```python
from build123d import *

# Parameters (mm, degrees)
F0_R      = 32.5
F1_DEPTH  = 196
F2_SIZE2  = 0.5
F2_SIZE   = 26
F3_R      = 32
F4_DEPTH  = 10
F5_R      = 26
F6_DEPTH  = 10
F7_R      = 7
F8_DEPTH  = 25
F9_R      = 9.5
F10_DEPTH = 10
F11_R     = 9
F12_DEPTH = 7


with BuildPart() as f1:
    # F0 (on Top) → F1 (new body)
    with BuildSketch(Plane.XY):
        Circle(F0_R)
    extrude(amount=F1_DEPTH)

    # F2
    f2_edges = [f1.edges().sort_by_distance(p)[0] for p in [
        (-32.5, 0, 196),
    ]]
    chamfer(f2_edges, length=F2_SIZE, length2=F2_SIZE2)

    # F3 (on face) → F4 (join)
    with BuildSketch(Plane(origin=(0, 0, 0), x_dir=(1, 0, 0), z_dir=(0, 0, -1))):
        Circle(F3_R)
    extrude(amount=F4_DEPTH)

    # F5 (on face) → F6 (join)
    with BuildSketch(Plane(origin=(0, 0, -10), x_dir=(1, 0, 0), z_dir=(0, 0, -1))):
        Circle(F5_R)
    extrude(amount=F6_DEPTH)

    # F7 (on face) → F8 (join)
    with BuildSketch(Plane(origin=(0, 0, -20), x_dir=(1, 0, 0), z_dir=(0, 0, -1))):
        Circle(F7_R)
    extrude(amount=F8_DEPTH)

    # F9 (on face) → F10 (join)
    with BuildSketch(Plane(origin=(0, 0, -45), x_dir=(1, 0, 0), z_dir=(0, 0, -1))):
        Circle(F9_R)
    extrude(amount=F10_DEPTH)

    # F11 (on face) → F12 (join)
    with BuildSketch(Plane.XY.offset(196)):
        Circle(F11_R)
    extrude(amount=F12_DEPTH)


solid = f1.part
```
Model file for the job. Use its own axes, mm. A direction names the side the tool comes from. Give positions to 0.01 mm unless a question says otherwise; leave off trailing zeros. Write each loop counter-clockwise with the first axis right and the second up, starting at its lowest first coordinate (ties: lowest second). Pieces come first, ordered by that corner, then holes. Notation, with made-up numbers: (25, -22.75) - (39, -22.75) arc R24 ccw to (39, 9.25) - close; hole circle Ø6 at (-1, 61.25). An arc over 180 degrees is marked (long way). One line per question, with ' | ' between items. Start each with the question number.
(1) Wall check: line 1 along Z through (x, y) = (-20.5, -10); line 2 along Z through (x, y) = (-1, 27); line 3 along X through (y, z) = (4, 154). Give the ranges that are in metal, low to high. Write a range as from..to.
(2) Slice it at A-A on z = 89. Write the cut outline in (x, y).
(3) Pin check, flat tips, straight feed: P1, Ø8, axis at y = -15, z = 116, coming from the -X side; P2, Ø1.5, axis at y = 18, z = 36.5, coming from the -X side; P3, Ø2, axis at x = 4.5, y = -11.5, coming from the -Z side. Stop position of each tip, or through.
(4) Two-plate mould, pull along Z, no slides. Class faces 1 (the face through (-32.215, 1.418, 183.182)), 2 (the face through (4.38, 8.43, -49.93)), 3 (the face through (6.466, 2.681, -32.325)): +Z half, -Z half, draft (parallel to the pull), parting line (faces both ways), or undercut.
(5) 3-axis set-ups, long thin cutter, end or side, ignore diameter. For faces 4 (the face through (7, -7, 196)), 5 (the face through (-4, 6, -45)), 6 (the face through (23.92, -21.52, 0)): which of +Z, -Z, +X, -X, +Y, -Y reach the whole face in a straight line?
Results below:
1) line 1: -20..196 | line 2: -10..196 | line 3: -32.25..32.25
2) outline: circle Ø65 at (0, 0)
3) P1: x = -30.58 | P2: x = -27.54 | P3: z = -20
4) face 1: +Z half | face 2: draft | face 3: undercut
5) face 4: +Z | face 5: none | face 6: -Z
